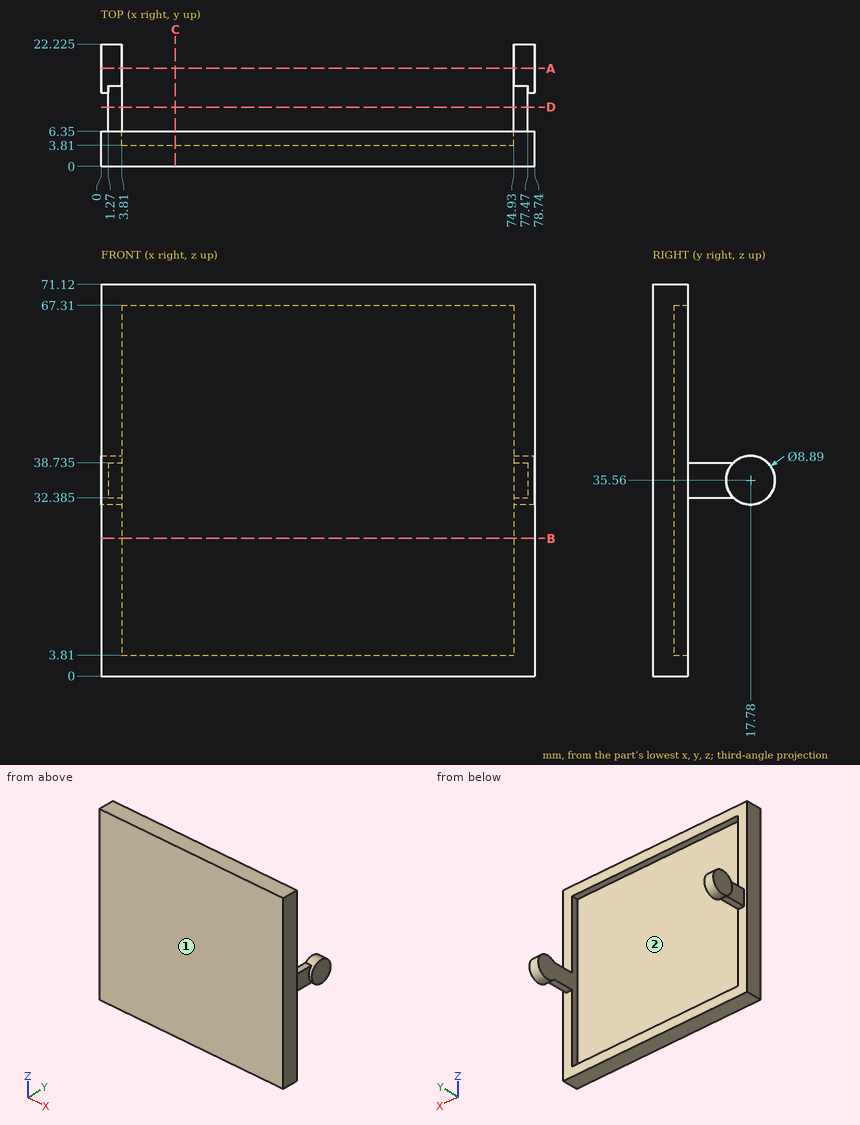
Print and shaded views of the part. All mm, measured from the part's lowest x, y and z. Round coordinates to 2 decimals unless told otherwise and drop trailing zeros. Write each loop counter-clockwise with the first axis right and the second up, starting at its lowest first coordinate (ties: lowest second). Pieces come first, ordered by that corner, then holes. Notation, with made-up numbers: (75, 63) - (83, 63) arc R30 cw to (83, 88) - close; hole circle Ø10 at (58.5, -20.5). An arc over 180 degrees is marked (long way). Write each question's results on one line, items separated by ' | '. Start each with the question number.
Item 1: Mould opens along Z. For the marked faces 1 and 2 say: pulls with the +Z half, pulls with the -Z half, needs draft (parallel to the pull), parting line crosses it, or undercut.
Item 2: Saw through at B-B (z = 25). Write the cut outline in (x, y), and give its area (3 significant figures).
Item 3: Saw through at D-D (y = 10.75). Write the cut outline in (x, z) (3 decimals), and give its area (3 significant figures).
Item 4: Saw through at C-C (x = 13.5). Write the cut outline in (y, z).
Item 5: Wall check: L1, parallel to X at y = 4.75, z = 13; L2, parallel to Z at x = 5, y = 5.75; L3, parallel to Y at x = 53, z = 49. Give the ranges that are in metal, low to high. Write a range as [from, to].
Item 6: Saw through at A-A (y = 17.78). Write the cut outline in (x, z) (3 decimals).
Item 7: Drop flat-ended pins along their axis: P1, Ø12, axis at y = 14, z = 56.5, coming from the -X side; P2, Ø1.9, axis at y = 12.5, z = 35.5, coming from the -X side; P3, Ø6, axis at x = 24.5, z = 37.5, coming from the +Y side; P4, Ø3, axis at y = 9.5, z = 34, coming from the +X side. Give the stop position or say it passes through.
Results are:
1) face 1: needs draft | face 2: undercut
2) outline: (0, 0) - (78.74, 0) - (78.74, 6.35) - (74.93, 6.35) - (74.93, 3.81) - (3.81, 3.81) - (3.81, 6.35) - (0, 6.35) - close | area: 319 mm²
3) outline: (1.27, 32.385) - (3.81, 32.385) - (3.81, 38.735) - (1.27, 38.735) - close; (74.93, 32.385) - (77.47, 32.385) - (77.47, 38.735) - (74.93, 38.735) - close | area: 32.3 mm²
4) outline: (0, 0) - (6.35, 0) - (6.35, 3.81) - (3.81, 3.81) - (3.81, 67.31) - (6.35, 67.31) - (6.35, 71.12) - (0, 71.12) - close
5) L1: x = [0, 3.81], [74.93, 78.74] | L2: z = [0, 3.81], [67.31, 71.12] | L3: y = [0, 3.81]
6) outline: (0, 31.115) - (3.81, 31.115) - (3.81, 40.005) - (0, 40.005) - close; (74.93, 31.115) - (78.74, 31.115) - (78.74, 40.005) - (74.93, 40.005) - close
7) P1: passes through | P2: stops at x = 0 | P3: stops at y = 3.81 | P4: stops at x = 77.47
